For this review, take the finished solid that the model builds, in its own axes (mm). Face numbers are marked on the shaded views. A direction names the side the tool comes from. Give positions to 0.01 mm unless a question says otherwise; leave off trailing zeros. Loops run counter-clockwise (first coordinate to the right, second up) from the corner with the lowest first, then second, coordinate; pieces in that order, holes last. Notation, with made-up numbers: (54.5, 83.25) - (78.5, 83.25) arc R15 cw to (78.5, 96.25) - close; hole circle Ø8 at (80.25, 67). An arc over 180 degrees is marked (long way). Answer as CSV lines item,"result".
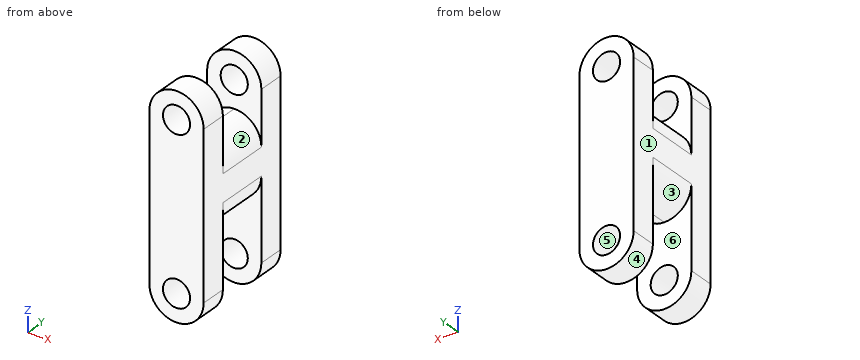
from build123d import *

# Parameters (mm, degrees)
SKETCH1_R           = 2.5
BOSS_EXTRUDE1_DEPTH = 20
SKETCH2_W           = 10
SKETCH2_H           = 10
CUT_EXTRUDE1_DEPTH  = 15
FILLET1_R           = 5
SKETCH3_W           = 10
SKETCH3_H           = 10
CUT_EXTRUDE3_DEPTH  = 10
FILLET3_R           = 5


with BuildPart() as part:
    # Sketch1 → Boss-Extrude1 (new body)
    with BuildSketch(Plane(origin=(0, 0, 0), x_dir=(1, 0, 0), z_dir=(0, 1, 0))):
        with BuildLine():
            Line((-5, 0), (-5, 30))
            ThreePointArc((-5, 30), (0, 35), (5, 30))
            Line((5, 30), (5, 0))
            ThreePointArc((5, 0), (0, -5), (-5, 0))
        make_face()
        with Locations(Location((0, 30, 0), (0, 0, 270))):
            Circle(SKETCH1_R, mode=Mode.SUBTRACT)
        with Locations(Location((0, 0, 0), (0, 0, 270))):
            Circle(SKETCH1_R, mode=Mode.SUBTRACT)
    extrude(amount=BOSS_EXTRUDE1_DEPTH)

    # Sketch2 → Cut-Extrude1 (cut)
    with BuildSketch(Plane(origin=(5, 0, 0), x_dir=(0, 0, -1), z_dir=(1, 0, 0))):
        with Locations((0, 10)):
            Rectangle(SKETCH2_W, SKETCH2_H)
    cut_extrude1 = extrude(amount=-CUT_EXTRUDE1_DEPTH, mode=Mode.SUBTRACT)

    # Mirror1: Cut-Extrude1 across plane
    add(cut_extrude1.mirror(Plane.XY.offset(-15)), mode=Mode.SUBTRACT)

    # Fillet1
    fillet1_edges = [part.edges().sort_by_distance(p)[0] for p in [
        (-5, 10, -25),
        (5, 10, -25),
        (-5, 10, -5),
        (5, 10, -5),
    ]]
    fillet(fillet1_edges, radius=FILLET1_R - 0.0001)  # a hair under: the kernel refuses the full size

    # Sketch3 → Cut-Extrude3 (cut)
    with BuildSketch(Plane(origin=(5, 0, 0), x_dir=(0, 0, -1), z_dir=(1, 0, 0))):
        with Locations((25, 10)):
            Rectangle(SKETCH3_W, SKETCH3_H)
    extrude(amount=-CUT_EXTRUDE3_DEPTH, mode=Mode.SUBTRACT)

    # Fillet3
    fillet3_edges = [part.edges().sort_by_distance(p)[0] for p in [
        (-5, 10, -20.0001),
        (5, 10, -20.0001),
    ]]
    fillet(fillet3_edges, radius=FILLET3_R - 0.0001)  # a hair under: the kernel refuses the full size


solid = part.part
1) Consider section D-D on z = -31. Write out the cut boundary in (x, y), and give its area (3 significant figures).
From the geometry:
outline,"(-4.9, 0) - (-2.29, 0) - (-2.29, 5) - (-4.9, 5) - close; (-4.9, 15) - (-2.29, 15) - (-2.29, 20) - (-4.9, 20) - close; (2.29, 0) - (4.9, 0) - (4.9, 5) - (2.29, 5) - close; (2.29, 15) - (4.9, 15) - (4.9, 20) - (2.29, 20) - close"
area,"52.2 mm^2"
2) Draft analysis for pull direction Z (two halves, no side actions). For the marked faces 4, 5 and 6, state which applies: pulls with the +Z half, pulls with the -Z half, needs draft (parallel to the pull), parting line crosses it, or undercut.
From the geometry:
face 4,"pulls with the -Z half"
face 5,"undercut"
face 6,"needs draft"
3) Wall thickness on line 1 (Z direction, x = 0, y = 2.45); line 2 (Y direction, x = 2.5, z = -33); line 3 (X direction, y = 4.05, z = -30): over which ranges is each line inside the solid? List them lowest first. Write a range as from..to.
From the geometry:
line 1,"z = -35..-32.5, -27.5..-2.5, 2.5..5"
line 2,"y = 0..5, 15..20"
line 3,"x = -5..-2.5, 2.5..5"
4) Machinability: for the marked faces 1, 2 and 3, which of the approach directions +Z, -Z, +X, -X, +Y, -Y give a long, thin tool a straight path to every point of the face, cutting with its end or side? Answer none if there is none.
From the geometry:
face 1,"+Z, -Z, -X, +Y, -Y"
face 2,"+Z, +X"
face 3,"-Z, -X"
5) Consider section C-C on x = -3. Write out the cut boundary in (y, z).
From the geometry:
outline,"(0, -34) - (5, -34) - (5, -19) - (15, -19) - (15, -34) - (20, -34) - (20, 4) - (15, 4) - (15, -6) - (5, -6) - (5, 4) - (0, 4) - close"
6) Consider section A-A on z = -22. Write out the cut boundary in (x, y), and give its area (3 significant figures).
From the geometry:
outline,"(-5, 0) - (5, 0) - (5, 5) - (-5, 5) - close; (-5, 15) - (5, 15) - (5, 20) - (-5, 20) - close"
area,"100 mm^2"
